```python
from build123d import *

# Parameters (mm, degrees)
CUT_EXTRUDE1_DEPTH      = 5
SKETCH3_R               = 27.671687605
CUT_EXTRUDE2_DEPTH      = 1.5
FILLET1_R               = 3
CUT_EXTRUDE3_DEPTH      = 11
CUT_EXTRUDE3_DEPTH_BACK = 1.5
SKETCH4_R               = 5.5


with BuildPart() as part:
    # Sketch1 → Revolve1 (revolve)
    with BuildSketch(Plane(origin=(0, 0, 0), x_dir=(0, 0, -1), z_dir=(1, 0, 0)), mode=Mode.PRIVATE) as revolve1_sk:
        Polygon((3, 31.471687605), (3, 4.5), (-3, 4.5), (-3, 31.471687605), (0, 29.587241701), align=None)
    revolve(revolve1_sk.sketch.rotate(Axis((0, 0, 0), (0, 0, -1)), 90), axis=Axis((0, 0, 0), (0, 0, -1)))

    # Sketch2 → Cut-Extrude1 (cut, symmetric)
    with BuildSketch(Plane.XY):
        with BuildLine():
            Line((-3, 27.307391304), (-3, 9.539392014))
            ThreePointArc((-3, 9.539392014), (-5.877852523, 8.090169944), (-8.145449953, 5.801003797))
            Line((-8.145449953, 5.801003797), (-25.04382146, 11.291617534))
            ThreePointArc((-25.04382146, 11.291617534), (-16.14745283, 22.225062136), (-3, 27.307391304))
        make_face()
        with BuildLine():
            Line((3, 27.307391304), (3, 9.539392014))
            ThreePointArc((3, 9.539392014), (5.877852523, 8.090169944), (8.145449953, 5.801003797))
            Line((8.145449953, 5.801003797), (25.04382146, 11.291617534))
            ThreePointArc((25.04382146, 11.291617534), (16.14745283, 22.225062136), (3, 27.307391304))
        make_face()
        with BuildLine():
            Line((26.897923426, 5.585278436), (9.99955192, 0.094664699))
            ThreePointArc((9.99955192, 0.094664699), (9.510565163, -3.090169944), (8.034164925, -5.954174499))
            Line((8.034164925, -5.954174499), (18.47793287, -20.328787881))
            ThreePointArc((18.47793287, -20.328787881), (26.12712751, -8.489218334), (26.897923426, 5.585278436))
        make_face()
        with BuildLine():
            Line((13.623830904, -23.855499394), (3.180062959, -9.480886012))
            ThreePointArc((3.180062959, -9.480886012), (0, -10), (-3.180062959, -9.480886012))
            Line((-3.180062959, -9.480886012), (-13.623830904, -23.855499394))
            ThreePointArc((-13.623830904, -23.855499394), (0, -27.471687605), (13.623830904, -23.855499394))
        make_face()
        with BuildLine():
            Line((-18.47793287, -20.328787881), (-8.034164925, -5.954174499))
            ThreePointArc((-8.034164925, -5.954174499), (-9.510565163, -3.090169944), (-9.99955192, 0.094664699))
            Line((-9.99955192, 0.094664699), (-26.897923426, 5.585278436))
            ThreePointArc((-26.897923426, 5.585278436), (-26.12712751, -8.489218334), (-18.47793287, -20.328787881))
        make_face()
    extrude(amount=CUT_EXTRUDE1_DEPTH, both=True, mode=Mode.SUBTRACT)

    # Sketch3 → Cut-Extrude2 (cut)
    with BuildSketch(Plane(origin=(0, 0, -3), x_dir=(-1, 0, 0), z_dir=(0, 0, -1))):
        Circle(SKETCH3_R)
    extrude(amount=-CUT_EXTRUDE2_DEPTH, mode=Mode.SUBTRACT)

    # Fillet1
    fillet1_edges = [part.edges().sort_by_distance(p)[0] for p in [
        (-8.034164925, -5.954174499, 0.75),
        (-18.47793287, -20.328787881, 0.75),
        (-9.99955192, 0.094664699, 0.75),
        (-26.897923426, 5.585278436, 0.75),
        (3.180062959, -9.480886012, 0.75),
        (13.623830904, -23.855499394, 0.75),
        (-3.180062959, -9.480886012, 0.75),
        (-13.623830904, -23.855499394, 0.75),
        (9.99955192, 0.094664699, 0.75),
        (26.897923426, 5.585278436, 0.75),
        (8.034164925, -5.954174499, 0.75),
        (18.47793287, -20.328787881, 0.75),
        (3, 9.539392014, 0.75),
        (3, 27.307391304, 0.75),
        (8.145449953, 5.801003797, 0.75),
        (25.04382146, 11.291617534, 0.75),
        (-8.145449953, 5.801003797, 0.75),
        (-25.04382146, 11.291617534, 0.75),
        (-3, 9.539392014, 0.75),
        (-3, 27.307391304, 0.75),
    ]]
    fillet(fillet1_edges, radius=FILLET1_R)

    # Sketch4 → Cut-Extrude3 (cut, two sides: drawn at the far end of the back side and taken through both)
    with BuildSketch(Plane(origin=(0, 0, 0), x_dir=(-1, 0, 0), z_dir=(0, 0, -1)).offset(-CUT_EXTRUDE3_DEPTH_BACK)):
        Circle(SKETCH4_R)
    extrude(amount=CUT_EXTRUDE3_DEPTH + CUT_EXTRUDE3_DEPTH_BACK, mode=Mode.SUBTRACT)


solid = part.part
```
The listing builds one solid part. Answer for the finished solid, in the listing's coordinates (mm). A direction names the side the tool comes from. Give positions to 0.01 mm unless a question says otherwise; leave off trailing zeros. Order: outer loops, then holes, each group sorted by start corner. A loop starts at its lowest first (then second) coordinate and runs counter-clockwise, first axis right, second up. Notation, with made-up numbers: (82, -13.5) -> (97, -13.5) arc R17 cw to (97, -1.5) -> close; hole circle Ø3 at (-34, 52). An arc over 180 degrees is marked (long way). Answer as CSV lines item,"result". Start each with the question number.
Q1. Determine the mould class of faces 3 (the cylindrical face through (23.543, 12.052, 0.719)), 4 (the flat face through (0, 28, -3)) for opening direction Y: pulls with the +Y half, pulls with the -Y half, needs draft (parallel to the pull), parting line crosses it, or undercut.
Q2. Which of the six approach directions +Z, -Z, +X, -X, +Y, -Y give full straight-line access (tool end or side, diameter ignored) to faces 1 (the cylindrical face through (18.738, -18.666, 0.719)), 2 (the flat face through (-6, 0, -1.5))?
Q3. A cutting plane is placed at A-A (x = 0). Determine the outline of the cut face in (y, z), then the cut area to 3 significant figures.
Q4. Find the intervals of material crossed by L1, parallel to X at y = 21.5, z = 1.15; L2, parallel to Y at x = 16.5, z = 0.3; L3, parallel to Y at x = -6, z = 1.2, in increasing order.
Q5. A cutting plane is placed at C-C (y = 8). Count the separate pieces of the cut face and the enclosed holes in it, then the cut area to 3 significant figures.
Q6. Given pin 1 (12 mm diameter, centred on x = 2.5, y = 2.5, fed in from -Z); pin 2 (8 mm diameter, centred on x = 0, y = 0, fed in from -Z); pin 3 (1.3 mm diameter, centred on y = 15.5, z = 1.5, fed in from +X); pin 4 (2 mm diameter, centred on y = 17.5, z = 1.5, fed in from -X), each flat-ended and moving along its own axis, determine where each tip first touches the part or whether it passes through.
Q7. A cutting plane is placed at B-B (z = -2.25). Determine the outline of the cut face in (x, y), then the cut area to 3 significant figures.
Results found:
1,face 3,"undercut"
1,face 4,"needs draft"
2,face 1,"+Z, -Z"
2,face 2,"-Z"
3,outline,"(-31.47, -3) -> (-27.67, -3) -> (-27.67, -1.5) -> (-27.47, -1.5) -> (-27.47, 3) -> (-31.47, 3) -> (-29.59, 0) -> close; (-10, -1.5) -> (-5.5, -1.5) -> (-5.5, 1.5) -> (-4.5, 1.5) -> (-4.5, 3) -> (-10, 3) -> close; (4.5, 1.5) -> (5.5, 1.5) -> (5.5, -1.5) -> (27.67, -1.5) -> (27.67, -3) -> (31.47, -3) -> (29.59, 0) -> (31.47, 3) -> (4.5, 3) -> close"
3,area,"158 mm2"
4,L1,"-21.36 to -17.1, -3 to 3, 17.1 to 21.36"
4,L2,"-24.79 to -17.59, 2.21 to 8.52, 21.96 to 24.79"
4,L3,"-29.74 to -26.81, -13.36 to 8, 26.72 to 29.74"
5,separate pieces,"3"
5,enclosed holes,"0"
5,area,"194 mm2"
6,pin 1,"z = -1.5"
6,pin 2,"through"
6,pin 3,"x = 26.9"
6,pin 4,"x = -26.03"
7,outline,"circle Ø62 at (0, 0); hole circle Ø55.34 at (0, 0)"
7,area,"614 mm2"
